Check sheet for the drawn part. Datum: minimum x, y, z corner. Units: mm. A direction names the side the tool comes from. Coordinates: 2 decimals unless noted, no trailing zeros. Order: outer loops, then holes, each group sorted by start corner. A loop starts at its lowest first (then second) coordinate and runs counter-clockwise, first axis right, second up. Notation, with made-up numbers: (-34, -18) - (-21, -18) arc R22 ccw to (-21, 8) - close; hole circle Ø5 at (-20, 19.5). An arc over 180 degrees is marked (long way). Put each result on its own line as item: value.
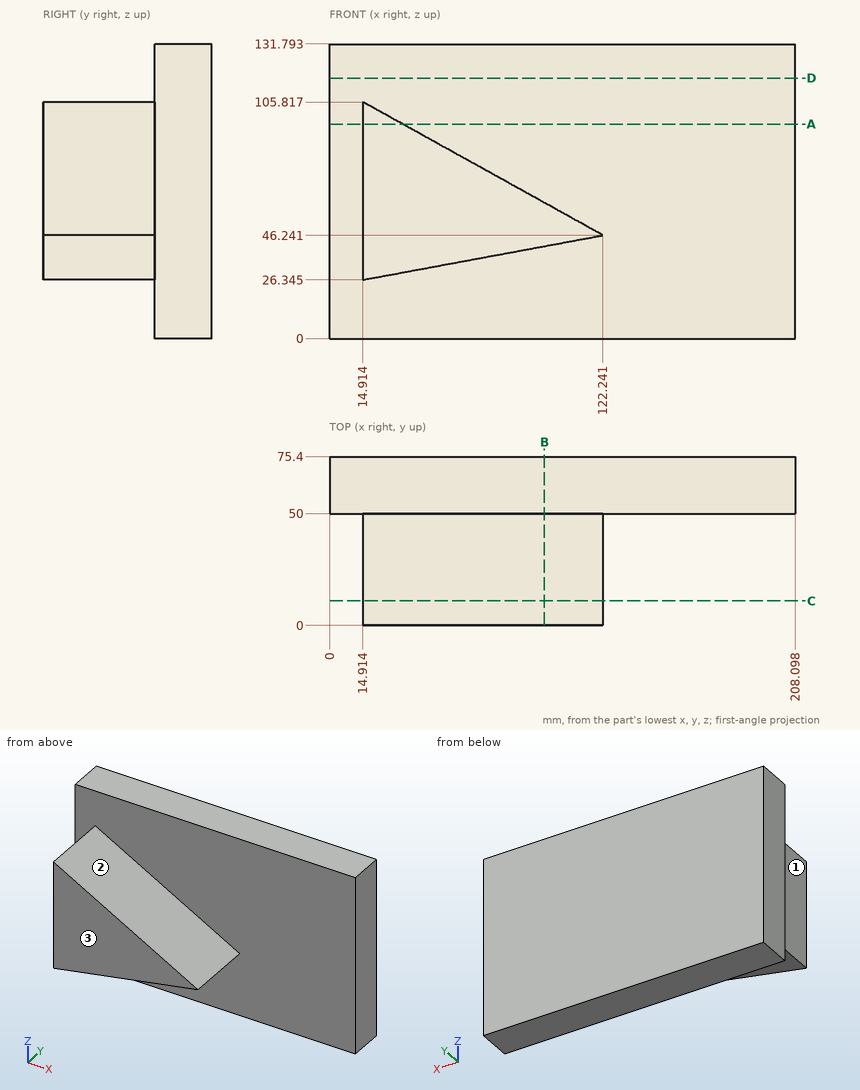
Q1. Section check B-B on x = 96. Record the boundary of the cut face in (y, z).
Answer block:
outline: (0, 41.38) - (50, 41.38) - (50, 0) - (75.4, 0) - (75.4, 131.79) - (50, 131.79) - (50, 60.81) - (0, 60.81) - close
Q2. Section check C-C on y = 11. Record the boundary of the cut face in (x, z) (1 decimal).
Answer block:
outline: (14.9, 26.3) - (122.2, 46.2) - (14.9, 105.8) - close
Q3. Section check A-A on z = 96. Record the boundary of the cut face in (x, y), then the cut area to 3 significant figures.
Answer block:
outline: (0, 50) - (14.91, 50) - (14.91, 0) - (32.6, 0) - (32.6, 50) - (208.1, 50) - (208.1, 75.4) - (0, 75.4) - close
area: 6,170 mm^2
Q4. Access from +Z, -Z, +X, -X, +Y, -Y to the whole of each face (thin tool, end or side, straight path). Record for the marked faces 1, 2 and 3.
Answer block:
face 1: +Z, -Z, -X, -Y
face 2: +Z, +X, -Y
face 3: +Z, -Z, +X, -X, -Y
Q5. Thickness scan on L1, parallel to Y at x = 183.5, z = 75; L2, parallel to Z at x = 28.5, y = 22 (1 decimal); L3, parallel to X at y = 9.5, z = 48 (1 decimal). Record the ranges inside material, lowest first. Write a range as [from, to].
Answer block:
L1: y = [50, 75.4]
L2: z = [28.9, 98.3]
L3: x = [14.9, 119.1]
Q6. Depth check by flat-ended pin: pin 1 Ø3 at (y, z) = (19.5, 50.5) entering from +X; pin 2 Ø1 at (y, z) = (42.5, 29) entering from -X; pin 3 Ø4 at (y, z) = (21.5, 107.5) entering from +X (1 decimal). Enter the tip coordinate at first touch or a pass-through.
Answer block:
pin 1: stops at x = 117.27
pin 2: stops at x = 14.91
pin 3: stops at x = 15.5
Q7. Section check D-D on z = 116.5. Record the boundary of the cut face in (x, y), then the cut area to 3 significant figures.
Answer block:
outline: (0, 50) - (208.1, 50) - (208.1, 75.4) - (0, 75.4) - close
area: 5,290 mm^2
